Geometry check sheet. Reference: the model listing, model coordinates, mm. A direction names the side the tool comes from. Round coordinates to 2 decimals unless told otherwise and drop trailing zeros. Answer as a JSON object with one key per item and string values. Group by question number.
```python
from build123d import *

# Parameters (mm, degrees)
CUT_EXTRUDE1_DEPTH = 0.75
FILLET1_R          = 0.125


with BuildPart() as part:
    # Sketch1 → Revolve1 (revolve)
    with BuildSketch(Plane(origin=(0, 0, 0), x_dir=(0, 0, -1), z_dir=(1, 0, 0))):
        with BuildLine():
            Line((0, 1.5), (-1.75, 1.5))
            ThreePointArc((-1.75, 1.5), (-2.334912942, 0.942930354), (-2.75, 0.25))
            Line((-2.75, 0.25), (-2.605662433, 0))
            Line((-2.605662433, 0), (-1.5, 0))
            Line((-1.5, 0), (-1.5, -12))
            Line((-1.5, -12), (0, -12))
            Line((0, -12), (0, 1.5))
        make_face()
    revolve(axis=Axis((0, -12, 0), (0, 1, 0)))

    # Sketch2 → Cut-Extrude1 (cut)
    with BuildSketch(Plane(origin=(0, 1.5, 0), x_dir=(1, 0, 0), z_dir=(0, 1, 0))):
        Polygon((0, 1.154700538), (-1, 0.577350269), (-1, -0.577350269), (0, -1.154700538), (1, -0.577350269), (1, 0.577350269), align=None)
    extrude(amount=-CUT_EXTRUDE1_DEPTH, mode=Mode.SUBTRACT)

    # Fillet1
    fillet1_edges = [part.edges().sort_by_distance(p)[0] for p in [
        (0.5, 1.5, -0.866025404),
        (-0.5, 1.5, -0.866025404),
        (-1, 1.5, 0),
        (-0.5, 1.5, 0.866025404),
        (0.5, 1.5, 0.866025404),
        (1, 1.5, 0),
        (0, 1.5, -1.75),
    ]]
    fillet(fillet1_edges, radius=FILLET1_R)


solid = part.part
```
1) Set-up check for faces 1 (the flat face through (-2, 0, 0)), 2 (the flat face through (0, -12, 0)): record each of +Z, -Z, +X, -X, +Y, -Y from which the full face is reachable in a straight line by a thin tool's end or side.
2) Thickness scan on line 1 along Y through (x, z) = (-0.95, 0.4); line 2 along X through (y, z) = (-7.5, -0.75); line 3 along Y through (x, z) = (-2, -1.75). Record the ranges inside material, lowest first. Write a range as [from, to].
3) Release check for a two-part mould opening along X. For faces 3 (the cylindrical face through (0.07, -6.08, -1.5)), 4 (the flat face through (0, 0.75, 0)), 5 (the flat face through (-1, 1.5, 1)) record: +X half, -X half, draft (parallel to the pull), parting line (faces both ways), or undercut.
4) Go/stop test with flat-tipped pins: P1, Ø0.6, axis at x = 0, z = -0.5, coming from the +Y side; P2, Ø0.5, axis at y = 1, z = 0, coming from the +X side; P3, Ø3, axis at y = -4.5, z = -0.5, coming from the -X side. Record where each tip stops, or that it passes through.
Final values:
{
 "1": {"face 1": "-Y", "face 2": "+Z, -Z, +X, -X, -Y"},
 "2": {"line 1": "y = [-12, 0.75]", "line 2": "x = [-1.3, 1.3]", "line 3": "y = [0.09, 0.45]"},
 "3": {"face 3": "parting line", "face 4": "undercut", "face 5": "draft"},
 "4": {"P1": "stops at y = 0.75", "P2": "stops at x = 2.48", "P3": "stops at x = -1.5"}
}
